Input: part model. Units: mm. Frame: model coordinates. Face numbers are marked on the shaded views. A direction names the side the tool comes from. Give positions to 0.01 mm unless a question says otherwise; leave off trailing zeros. Loops run counter-clockwise (first coordinate to the right, second up) from the corner with the lowest first, then second, coordinate; pieces in that order, holes last. Notation, with made-up numbers: (-39.5, 31.5) - (-4.5, 31.5) arc R29 ccw to (-4.5, 53.5) - close; hole circle Ø3 at (-34, -32). An arc over 180 degrees is marked (long way). Answer as a JSON object with one key per item and string values. Group by question number.
(1) Material intervals for L1, parallel to Z at x = 0, y = -2.5; L2, parallel to Y at x = 11, z = 0.5 (3 decimals); L3, parallel to Z at x = -2.5, y = -0.75, sorted ascending.
(2) Access query for the marked faces 4, 5 and 6. Directions: +Z, -Z, +X, -X, +Y, -Y. A direction counts if a zero-diameter tool reaches every point of the face in a straight line with its end or side. Return the directions, or none.
(3) Pin query (flat end, axial travel): P1, Ø3, axis at x = -8, y = -0.5, coming from the +Z side; P2, Ø1.5, axis at y = -1.5, z = -7, coming from the +X side; P3, Ø1.5, axis at y = 0, z = 3, coming from the -X side; P4, Ø2.5, axis at x = 0, z = 0, coming from the +Y side. Return the tip coordinate at first contact, or that it passes through.
(4) Mould query, pull axis Z, two halves, no side actions, for the marked faces 1, 2 and 3. Classes: +Z half, -Z half, draft (parallel to the pull), parting line (faces both ways), or undercut.
(5) Section query A-A (y = -0.5). Return loops of the section in (x, z) (3 decimals), plus the area to 3 significant figures.
(6) Section query B-B (z = 0). Return loops of the section in (x, y) (3 decimals).
(7) Section query C-C (y = 2.5). Return loops of the section in (x, z).
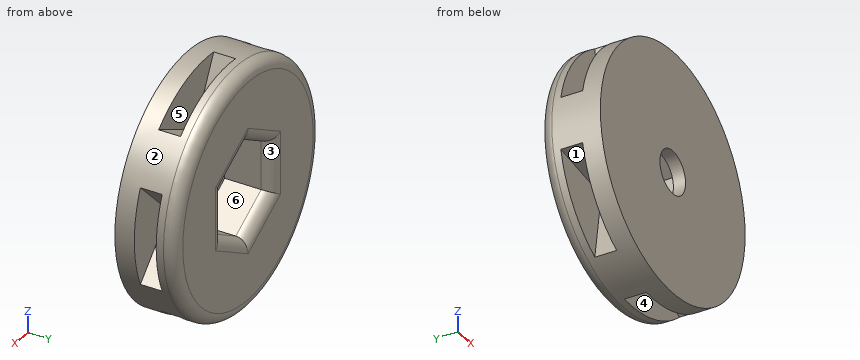
```python
from build123d import *

# Parameters (mm, degrees)
SKETCH2_R            = 12.7
BOSS_EXTRUDE1_DEPTH  = 3.175
CUT_EXTRUDE1_DEPTH   = 1.143
CIRPATTERN1_COUNT    = 5
FILLET1_R            = 1.27
BOSS_EXTRUDE2_DEPTH  = 1.27
M4_CLEARANCE_HOLE1_D = 4.5


with BuildPart() as part:
    # Sketch2 → Boss-Extrude1 (new body, symmetric)
    with BuildSketch(Plane(origin=(0, 0, 0), x_dir=(1, 0, 0), z_dir=(0, 1, 0))):
        Circle(SKETCH2_R)
        Polygon((0, 5.132643893), (-4.445, 2.566321947), (-4.445, -2.566321947), (0, -5.132643893), (4.445, -2.566321947), (4.445, 2.566321947), align=None, mode=Mode.SUBTRACT)
    extrude(amount=BOSS_EXTRUDE1_DEPTH, both=True)

    # Sketch3 → Cut-Extrude1 (cut, symmetric)
    with BuildSketch(Plane(origin=(0, 0, 0), x_dir=(1, 0, 0), z_dir=(0, 1, 0))):
        with BuildLine():
            Line((11.639742265, 5.08), (7.829742265, 1.27))
            Line((7.829742265, 1.27), (7.829742265, -1.27))
            Line((7.829742265, -1.27), (11.639742265, -5.08))
            ThreePointArc((11.639742265, -5.08), (12.7, 0), (11.639742265, 5.08))
        make_face()
    cut_extrude1 = extrude(amount=CUT_EXTRUDE1_DEPTH, both=True, mode=Mode.SUBTRACT)

    # CirPattern1: Cut-Extrude1 ×5 about axis
    cirpattern1_axis = Axis((0, 0, 0), (0, 1, 0))
    for i in range(1, CIRPATTERN1_COUNT):
        add(cut_extrude1.rotate(cirpattern1_axis, i * 360 / CIRPATTERN1_COUNT), mode=Mode.SUBTRACT)

    # Fillet1
    fillet1_edges = [part.edges().sort_by_distance(p)[0] for p in [
        (2.2225, 3.175, -3.84948292),
        (-2.2225, 3.175, -3.84948292),
        (-4.445, 3.175, 0),
        (-2.2225, 3.175, 3.84948292),
        (2.2225, 3.175, 3.84948292),
        (4.445, 3.175, 0),
        (-12.7, 3.175, 0),
    ]]
    fillet(fillet1_edges, radius=FILLET1_R)

    # Sketch4 → Boss-Extrude2 (add)
    with BuildSketch(Plane.XZ.offset(3.175)):
        Polygon((4.445, 2.566321947), (4.445, -2.566321947), (0, -5.132643893), (-4.445, -2.566321947), (-4.445, 2.566321947), (0, 5.132643893), align=None)
    extrude(amount=-BOSS_EXTRUDE2_DEPTH)

    # M4 Clearance Hole1 (through all)
    with Locations(Plane(origin=(0, -1.905, 0), x_dir=(1, 0, 0), z_dir=(0, 1, 0))):
        with Locations((0, 0)):
            Hole(M4_CLEARANCE_HOLE1_D / 2)


solid = part.part
```
Recorded:
{
 "1": {"L1": "z = -12.7 to -2.25, 2.25 to 12.7", "L2": "y = -3.175 to -1.143, 1.143 to 3.175", "L3": "z = -12.45 to -3.69, 3.69 to 12.45"},
 "2": {"face 4": "-Z", "face 5": "+Z", "face 6": "+Y"},
 "3": {"P1": "stops at z = 10.82", "P2": "stops at x = 11.06", "P3": "stops at x = -12.5", "P4": "passes through"},
 "4": {"face 1": "-Z half", "face 2": "parting line", "face 3": "undercut"},
 "5": {"outline": "(-12.403, -2.732) - (-7.081, -3.575) - (-5.588, -5.63) - (-6.431, -10.951) arc R12.7 ccw to (-1.234, -12.64) - (1.212, -7.839) - (3.627, -7.054) - (8.428, -9.5) arc R12.7 ccw to (11.64, -5.08) - (7.83, -1.27) - (7.83, 1.27) - (11.64, 5.08) arc R12.7 ccw to (8.428, 9.5) - (3.627, 7.054) - (1.212, 7.839) - (-1.234, 12.64) arc R12.7 ccw to (-6.431, 10.951) - (-5.588, 5.63) - (-7.081, 3.575) - (-12.403, 2.732) arc R12.7 ccw to start; hole (-4.445, -2.566) - (0, -5.133) - (4.445, -2.566) - (4.445, 2.566) - (0, 5.133) - (-4.445, 2.566) - close", "area": "281 mm^2"},
 "6": {"outline": "(-12.7, -3.175) - (-2.25, -3.175) - (-2.25, -1.905) - (-4.445, -1.905) - (-4.445, 1.905) arc R1.27 ccw to (-5.715, 3.175) - (-11.43, 3.175) arc R1.27 ccw to (-12.7, 1.905) - close; (2.25, -3.175) - (12.7, -3.175) - (12.7, -1.143) - (7.83, -1.143) - (7.83, 1.143) - (12.7, 1.143) - (12.7, 1.905) arc R1.27 ccw to (11.43, 3.175) - (5.715, 3.175) arc R1.27 ccw to (4.445, 1.905) - (4.445, -1.905) - (2.25, -1.905) - close"},
 "7": {"outline": "circle Ø25.1 at (0, 0); hole (-4.59, -2.65) - (0, -5.3) - (4.59, -2.65) - (4.59, 2.65) - (0, 5.3) - (-4.59, 2.65) - close"}
}
